For this review, take the finished solid that the model builds, in its own axes (mm). A direction names the side the tool comes from. Coordinates: 2 decimals unless noted, no trailing zeros. Loops run counter-clockwise (first coordinate to the right, second up) from the corner with the lowest first, then second, coordinate; pieces in that order, holes last. Notation, with made-up numbers: (-11, -8.5) -> (35, -8.5) arc R24 ccw to (35, 3.5) -> close; hole circle Ø3 at (2.25, 17.5). An arc over 180 degrees is marked (long way). Answer in a Markdown table with one row per item.
from build123d import *

# Parameters (mm, degrees)
F2_R     = 5
F3_R     = 1.5
F4_DEPTH = 70.5


with BuildPart() as f1:
    # F0 (on Top) → F1 (revolve)
    with BuildSketch(Plane.XY):
        Polygon((0, -40), (0, 0), (-15, 0), (-15, -20), (-36.239058, -20), (-36.239058, -40), align=None)
    revolve(axis=Axis((0, -11.717667, 0), (0, -1, 0)))

    # F2
    f2_edges = [f1.edges().sort_by_distance(p)[0] for p in [
        (15, 0, 0),
        (36.239058, -20, 0),
        (36.239058, -40, 0),
    ]]
    fillet(f2_edges, radius=F2_R)

    # F3 (on face) → F4 (cut)
    with BuildSketch(Plane.XZ.offset(40)):
        Circle(F3_R)
    extrude(amount=-F4_DEPTH, mode=Mode.SUBTRACT)


solid = f1.part
Item 1: Take a section at B-B, the plane z = 0. State the section outline as (x, y) points.
Worked answers:
| item | result |
|---|---|
| outline | (-36.24, -35) arc R5 ccw to (-31.24, -40) -> (-1.5, -40) -> (-1.5, 0) -> (-10, 0) arc R5 ccw to (-15, -5) -> (-15, -20) -> (-31.24, -20) arc R5 ccw to (-36.24, -25) -> close; (1.5, -40) -> (31.24, -40) arc R5 ccw to (36.24, -35) -> (36.24, -25) arc R5 ccw to (31.24, -20) -> (15, -20) -> (15, -5) arc R5 ccw to (10, 0) -> (1.5, 0) -> close |
Item 2: Take a section at D-D, the plane y = -7. State the section outline as (x, z) points.
Worked answers:
| item | result |
|---|---|
| outline | circle Ø30 at (0, 0); hole circle Ø3 at (0, 0) |
Item 3: For L1, parallel to Z at x = 0, y = -13.5; L2, parallel to Z at x = 0, y = -29; L3, parallel to Y at x = 2, z = -31, list the stretches that pass through material, from the lowest coordinate up.
Worked answers:
| item | result |
|---|---|
| L1 | -15 to -1.5, 1.5 to 15 |
| L2 | -36.24 to -1.5, 1.5 to 36.24 |
| L3 | -40 to -20 |
Item 4: Take a section at C-C, the plane y = -32.5. State the section outline as (x, z) points, and give its area (3 significant figures).
Worked answers:
| item | result |
|---|---|
| outline | circle Ø72.48 at (0, 0); hole circle Ø3 at (0, 0) |
| area | 4,120 mm² |
Item 5: Take a section at A-A, the plane x = 0. State the section outline as (y, z) points, and give its area (3 significant figures).
Worked answers:
| item | result |
|---|---|
| outline | (-40, -31.24) arc R5 ccw to (-35, -36.24) -> (-25, -36.24) arc R5 ccw to (-20, -31.24) -> (-20, -15) -> (-5, -15) arc R5 ccw to (0, -10) -> (0, -1.5) -> (-40, -1.5) -> close; (-40, 1.5) -> (0, 1.5) -> (0, 10) arc R5 ccw to (-5, 15) -> (-20, 15) -> (-20, 31.24) arc R5 ccw to (-25, 36.24) -> (-35, 36.24) arc R5 ccw to (-40, 31.24) -> close |
| area | 1,900 mm² |
Item 6: Insertion check: pin 1 (4 mm diameter, centred on x = 23.5, z = -6, fed in from +Y); pin 2 (2 mm diameter, centred on y = -24, z = 23, fed in from -X); pin 3 (12 mm diameter, centred on x = -12, y = -33.5, fed in from +Z). Each pin has a flat end and moves straight along its axis. Give the tip position at first contact, or say it passes through.
Worked answers:
| item | result |
|---|---|
| pin 1 | y = -20 |
| pin 2 | x = -28.7 |
| pin 3 | z = 35.74 |
Item 7: For faces 1 (the flat face through (13.4, -20, -7.4)), 2 (the flat face through (2, 0, 0)), list the 3-axis set-ups (+Z, -Z, +X, -X, +Y, -Y) from which the entire face can be reached by the end or side of a thin tool; tool diameter is ignored.
Worked answers:
| item | result |
|---|---|
| face 1 | +Y |
| face 2 | +Z, -Z, +X, -X, +Y |
Item 8: The part is to be moulded in two halves that separate along X. For faces 3 (the cylindrical face through (4.72, -30.07, -35.93)), 4 (the flat face through (-7, -40, 0)), 5 (the cylindrical face through (-1.5, -20.28, 0.07)), say which applies: +X half, -X half, draft (parallel to the pull), parting line (faces both ways), or undercut.
Worked answers:
| item | result |
|---|---|
| face 3 | parting line |
| face 4 | draft |
| face 5 | undercut |
